Build history of the part. All positions in model axes, mm. Coordinates: 2 decimals unless noted, no trailing zeros. Write each question's results on one line, items separated by ' | '. Start each with the question number.
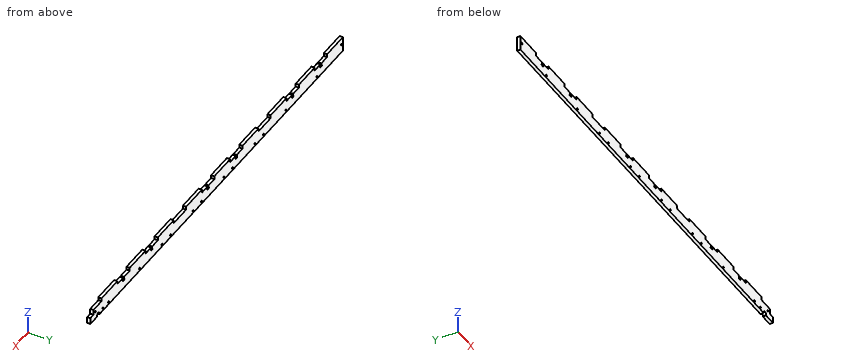
from build123d import *

# Parameters (mm, degrees)
DODANIE_WYCI_GNI_CIE2_DEPTH      = 3
DODANIE_WYCI_GNI_CIE2_DEPTH_BACK = 3
SZKIC1_W                         = 880
SZKIC1_H                         = 69
SZKIC1_W_2                       = 735
SZKIC1_H_2                       = 28
SZKIC2_W                         = 40
SZKIC2_H                         = 6
WYTNIJ_WYCI_GNI_CIE1_DEPTH       = 6
SZYK_LINIOWY1_COUNT              = 13
SZYK_LINIOWY1_PITCH              = 91
WYTNIJ_WYCI_GNI_CIE2_DEPTH       = 6
SZKIC9_R                         = 12.5
WYTNIJ_WYCI_GNI_CIE6_DEPTH       = 6
WYTNIJ_WYCI_GNI_CIE7_DEPTH       = 6
SZKIC13_W                        = 25
SZKIC13_H                        = 15
WYTNIJ_WYCI_GNI_CIE8_DEPTH       = 6
SZYK_LINIOWY3_COUNT              = 2
SZYK_LINIOWY3_PITCH              = 91
SZYK_LINIOWY3_COUNT_DIR2         = 3
SZYK_LINIOWY3_PITCH_DIR2         = 273
SZKIC14_OUTSIDE_W                = 1058.544
SZKIC14_OUTSIDE_H                = 247.544
SZKIC14_OUTSIDE_W_2              = 815
SZKIC14_OUTSIDE_H_2              = 28
WYTNIJ_WYCI_GNI_CIE9_DEPTH       = 10
SZKIC15_R                        = 1.55
WYTNIJ_WYCI_GNI_CIE10_DEPTH      = 10
SZKIC18_R                        = 1.55
WYTNIJ_WYCI_GNI_CIE11_DEPTH      = 10
SZKIC19_R                        = 1.55
WYTNIJ_WYCI_GNI_CIE12_DEPTH      = 10
SZYK_LINIOWY4_COUNT              = 6
SZYK_LINIOWY4_PITCH              = 100
SZKIC20_W                        = 10
SZKIC20_H                        = 10
WYTNIJ_WYCI_GNI_CIE13_DEPTH      = 10


with BuildPart() as part:
    # Szkic1 → Dodanie-wyci_gni_cie2 (new, two sides: drawn at the far end of the back side and taken through both)
    with BuildSketch(Plane(origin=(0, -418.87633849, -418.87633849), x_dir=(1, 0, 0), z_dir=(0, 1, 0)).offset(-DODANIE_WYCI_GNI_CIE2_DEPTH_BACK)):
        with Locations((-705.368459045, -443.37633849)):
            Rectangle(SZKIC1_W, SZKIC1_H)
        with Locations((-703.368459045, -435.87633849)):
            Rectangle(SZKIC1_W_2, SZKIC1_H_2, mode=Mode.SUBTRACT)
    extrude(amount=DODANIE_WYCI_GNI_CIE2_DEPTH + DODANIE_WYCI_GNI_CIE2_DEPTH_BACK)

    # Szkic2 → Wytnij-wyci_gni_cie1 (cut)
    with BuildSketch(Plane.XY.offset(59)):
        with Locations((-1125.368459045, -418.87633849)):
            Rectangle(SZKIC2_W, SZKIC2_H)
    wytnij_wyci_gni_cie1 = extrude(amount=-WYTNIJ_WYCI_GNI_CIE1_DEPTH, mode=Mode.SUBTRACT)

    # Szyk liniowy1: Wytnij-wyci_gni_cie1 ×13
    with Locations(*[(i * SZYK_LINIOWY1_PITCH, 0, 0) for i in range(1, SZYK_LINIOWY1_COUNT)]):
        add(wytnij_wyci_gni_cie1, mode=Mode.SUBTRACT)

    # Szkic3 → Wytnij-wyci_gni_cie2 (cut)
    with BuildSketch(Plane(origin=(0, -415.87633849, 0), x_dir=(1, 0, 0), z_dir=(0, 1, 0))):
        Polygon((-1032.818459045, -53), (-1035.918459045, -53), (-1035.918459045, -49), (-1037.293459045, -49), (-1037.293459045, -47), (-1035.918459045, -47), (-1035.918459045, -46.5), (-1032.818459045, -46.5), (-1032.818459045, -47), (-1031.443459045, -47), (-1031.443459045, -49), (-1032.818459045, -49), align=None)
    wytnij_wyci_gni_cie2 = extrude(amount=-WYTNIJ_WYCI_GNI_CIE2_DEPTH, mode=Mode.SUBTRACT)

    # Szkic9 → Wytnij-wyci_gni_cie6 (cut)
    with BuildSketch(Plane(origin=(0, -415.87633849, 0), x_dir=(1, 0, 0), z_dir=(0, 1, 0))):
        with Locations(Location((-300.706340265, -17.43, 0), (0, 0, 180))):
            Circle(SZKIC9_R)
    extrude(amount=-WYTNIJ_WYCI_GNI_CIE6_DEPTH, mode=Mode.SUBTRACT)

    # Szkic11 → Wytnij-wyci_gni_cie7 (cut)
    with BuildSketch(Plane.XZ.offset(421.87633849)):
        with BuildLine():
            Line((-319.956340265, 32.93), (-319.956340265, 30.976099153))
            Line((-319.956340265, 30.976099153), (-312.456340265, 30.976099153))
            Line((-312.456340265, 30.976099153), (-312.456340265, 32.93))
            ThreePointArc((-312.456340265, 32.93), (-316.206340265, 36.68), (-319.956340265, 32.93))
        make_face()
    extrude(amount=-WYTNIJ_WYCI_GNI_CIE7_DEPTH, mode=Mode.SUBTRACT)

    # Szkic13 → Wytnij-wyci_gni_cie8 (cut)
    with BuildSketch(Plane(origin=(0, -415.87633849, 0), x_dir=(1, 0, 0), z_dir=(0, 1, 0))):
        with Locations((-277.868459045, -51.5)):
            Rectangle(SZKIC13_W, SZKIC13_H)
    extrude(amount=-WYTNIJ_WYCI_GNI_CIE8_DEPTH, mode=Mode.SUBTRACT)

    # Szyk liniowy3: Wytnij-wyci_gni_cie2 2 × 3
    with Locations(*[Vector(1, 0, 0) * (i * SZYK_LINIOWY3_PITCH) + Vector(1, 0, 0) * (j * SZYK_LINIOWY3_PITCH_DIR2) for i in range(SZYK_LINIOWY3_COUNT) for j in range(SZYK_LINIOWY3_COUNT_DIR2) if (i, j) != (0, 0)]):
        add(wytnij_wyci_gni_cie2, mode=Mode.SUBTRACT)

    # Szkic14 outside → Wytnij-wyci_gni_cie9 (cut)
    with BuildSketch(Plane(origin=(0, -415.87633849, 0), x_dir=(1, 0, 0), z_dir=(0, 1, 0))):
        with Locations((-705.368, -24.5)):
            Rectangle(SZKIC14_OUTSIDE_W, SZKIC14_OUTSIDE_H)
        with Locations((-697.868459045, -45)):
            Rectangle(SZKIC14_OUTSIDE_W_2, SZKIC14_OUTSIDE_H_2, mode=Mode.SUBTRACT)
    extrude(amount=-WYTNIJ_WYCI_GNI_CIE9_DEPTH, mode=Mode.SUBTRACT)

    # Szkic15 → Wytnij-wyci_gni_cie10 (cut)
    with BuildSketch(Plane(origin=(0, -415.87633849, 0), x_dir=(1, 0, 0), z_dir=(0, 1, 0))):
        with Locations(Location((-1100.368459045, -47, 0), (0, 0, 180))):
            Circle(SZKIC15_R)
        with Locations(Location((-306.36620557, -45, 0), (0, 0, 180))):
            Circle(SZKIC15_R)
    extrude(amount=-WYTNIJ_WYCI_GNI_CIE10_DEPTH, mode=Mode.SUBTRACT)

    # Szkic18 → Wytnij-wyci_gni_cie11 (cut)
    with BuildSketch(Plane(origin=(0, -415.87633849, 0), x_dir=(1, 0, 0), z_dir=(0, 1, 0))):
        with Locations(Location((-330.638459045, -35.5, 0), (0, 0, 180))):
            Circle(SZKIC18_R)
    extrude(amount=-WYTNIJ_WYCI_GNI_CIE11_DEPTH, mode=Mode.SUBTRACT)

    # Szkic19 → Wytnij-wyci_gni_cie12 (cut)
    with BuildSketch(Plane(origin=(0, -415.87633849, 0), x_dir=(1, 0, 0), z_dir=(0, 1, 0))):
        with Locations(Location((-1021.368458991, -35.5, 0), (0, 0, 180))):
            Circle(SZKIC19_R)
        with Locations(Location((-849.218458991, -35.5, 0), (0, 0, 180))):
            Circle(SZKIC19_R)
    wytnij_wyci_gni_cie12 = extrude(amount=-WYTNIJ_WYCI_GNI_CIE12_DEPTH, mode=Mode.SUBTRACT)

    # Szyk liniowy4: Wytnij-wyci_gni_cie12 ×6
    with Locations(*[(i * SZYK_LINIOWY4_PITCH, 0, 0) for i in range(1, SZYK_LINIOWY4_COUNT)]):
        add(wytnij_wyci_gni_cie12, mode=Mode.SUBTRACT)

    # Szkic20 → Wytnij-wyci_gni_cie13 (cut)
    with BuildSketch(Plane(origin=(0, -415.87633849, 0), x_dir=(1, 0, 0), z_dir=(0, 1, 0))):
        with Locations((-295.368459045, -48)):
            Rectangle(SZKIC20_W, SZKIC20_H)
    extrude(amount=-WYTNIJ_WYCI_GNI_CIE13_DEPTH, mode=Mode.SUBTRACT)


solid = part.part
1. Wall check: line 1 along Z through (x, y) = (-522, -417.5); line 2 along X through (y, z) = (-417.25, 44.5); line 3 along Z through (x, y) = (-406.5, -418.95). Give the ranges that are in metal, low to high.
2. Pin check, flat tips, straight feed: pin 1 (1 mm diameter, centred on x = -767.5, y = -418, fed in from +Z); pin 2 (0.6 mm diameter, centred on y = -418, z = 47, fed in from +X). Stop position of each tip, or through.
3. Band-saw the part on A-A, the plane y = -417.25. Give the number of separate pieces and of enclosed holes in the cut face, plus the area to 3 significant figures.
Checked values:
1) line 1: 31 to 34.08, 36.92 to 59 | line 2: -1105.37 to -307.83, -304.9 to -300.37 | line 3: 31 to 53
2) pin 1: z = 53 | pin 2: x = -300.37
3) separate pieces: 1 | enclosed holes: 15 | area: 20,300 mm²
